Here's how the part is built. I have some questions about the finished solid (model axes, mm). Face numbers are marked on the shaded views. A direction names the side the tool comes from. Coordinates: 2 decimals unless noted, no trailing zeros. Write each loop counter-clockwise with the first axis right and the second up, starting at its lowest first coordinate (ties: lowest second). Pieces come first, ordered by that corner, then holes.
```python
from build123d import *

# Parameters (mm, degrees)
ESQUISSE1_R                        = 52
ESQUISSE1_R_2                      = 7
BOSS_EXTRU_1_DEPTH                 = 20
ESQUISSE2_W                        = 50
ESQUISSE2_H                        = 10
BOSS_EXTRU_2_DEPTH                 = 60
CONG_1_R                           = 25
ESQUISSE3_R                        = 6
ENL_V_MAT_EXTRU_1_DEPTH            = 40
R_P_TITION_CIRCULAIRE1_COUNT       = 2
CONG_1_OF_R_P_TITION_CIRCULAIRE1_R = 25
ESQUISSE5_R                        = 1.6
ENL_V_MAT_EXTRU_2_DEPTH            = 20
R_P_TITION_CIRCULAIRE2_COUNT       = 6
ESQUISSE6_R                        = 3
ENL_V_MAT_EXTRU_3_DEPTH            = 9
ENL_V_START                        = -10
ESQUISSE7_W                        = 80.1
ESQUISSE7_H                        = 5
ENL_V_MAT_EXTRU_4_DEPTH            = 45


with BuildPart() as part:
    # Esquisse1 → Boss.-Extru.1 (new body)
    with BuildSketch(Plane(origin=(0, 0, 0), x_dir=(1, 0, 0), z_dir=(0, 1, 0))):
        with Locations(Location((0, 0, 0), (0, 0, 270))):
            Circle(ESQUISSE1_R)
        with Locations(Location((0, 0, 0), (0, 0, 270))):
            Circle(ESQUISSE1_R_2, mode=Mode.SUBTRACT)
    extrude(amount=BOSS_EXTRU_1_DEPTH)

    # Esquisse2 → Boss.-Extru.2 (add)
    with BuildSketch(Plane(origin=(0, 20, 0), x_dir=(1, 0, 0), z_dir=(0, 1, 0))):
        with Locations((0, 25)):
            Rectangle(ESQUISSE2_W, ESQUISSE2_H)
    boss_extru_2 = extrude(amount=BOSS_EXTRU_2_DEPTH)

    # Congé1
    cong_1_edges = [part.edges().sort_by_distance(p)[0] for p in [
        (25, 80, -25),
        (-25, 80, -25),
    ]]
    fillet(cong_1_edges, radius=CONG_1_R - 0.0001)  # a hair under: the kernel refuses the full size

    # Esquisse3 → Enlèv. mat.-Extru.1 (cut)
    with BuildSketch(Plane(origin=(0, 0, -30), x_dir=(-1, 0, 0), z_dir=(0, 0, -1))):
        with Locations((0, 64)):
            Circle(ESQUISSE3_R)
    enl_v_mat_extru_1 = extrude(amount=-ENL_V_MAT_EXTRU_1_DEPTH, mode=Mode.SUBTRACT)

    # Répétition circulaire1: Boss.-Extru.2, Enlèv. mat.-Extru.1 ×2 about axis
    r_p_tition_circulaire1_axis = Axis((0, 0, 0), (0, 1, 0))
    add([boss_extru_2.rotate(r_p_tition_circulaire1_axis, i * 360 / R_P_TITION_CIRCULAIRE1_COUNT) for i in range(1, R_P_TITION_CIRCULAIRE1_COUNT)])
    add([enl_v_mat_extru_1.rotate(r_p_tition_circulaire1_axis, i * 360 / R_P_TITION_CIRCULAIRE1_COUNT) for i in range(1, R_P_TITION_CIRCULAIRE1_COUNT)], mode=Mode.SUBTRACT)

    # Congé1 of Répétition circulaire1
    cong_1_of_r_p_tition_circulaire1_edges = [part.edges().sort_by_distance(p)[0] for p in [
        (-25, 80, 25),
        (25, 80, 25),
    ]]
    fillet(cong_1_of_r_p_tition_circulaire1_edges, radius=CONG_1_OF_R_P_TITION_CIRCULAIRE1_R - 0.0001)  # a hair under: the kernel refuses the full size

    # Esquisse5 → Enlèv. mat.-Extru.2 (cut)
    with BuildSketch(Plane.XZ):
        with Locations(Location((0, 35, 0), (0, 0, 270))):
            Circle(ESQUISSE5_R)
    enl_v_mat_extru_2 = extrude(amount=-ENL_V_MAT_EXTRU_2_DEPTH, mode=Mode.SUBTRACT)

    # Répétition circulaire2: Enlèv. mat.-Extru.2 ×6 about axis
    r_p_tition_circulaire2_axis = Axis((0, 0, 0), (0, 1, 0))
    for i in range(1, R_P_TITION_CIRCULAIRE2_COUNT):
        add(enl_v_mat_extru_2.rotate(r_p_tition_circulaire2_axis, i * 360 / R_P_TITION_CIRCULAIRE2_COUNT), mode=Mode.SUBTRACT)

    # Esquisse6 → Enlèv. mat.-Extru.3 (cut)
    with BuildSketch(Plane(origin=(0, 20, 0), x_dir=(1, 0, 0), z_dir=(0, 1, 0))):
        with Locations(Location((30.310889132, 17.5, 0), (0, 0, 270))):
            Circle(ESQUISSE6_R)
        with Locations(Location((30.310889132, -17.5, 0), (0, 0, 270))):
            Circle(ESQUISSE6_R)
        with Locations(Location((0, -35, 0), (0, 0, 270))):
            Circle(ESQUISSE6_R)
        with Locations(Location((-30.310889132, -17.5, 0), (0, 0, 270))):
            Circle(ESQUISSE6_R)
        with Locations(Location((-30.310889132, 17.5, 0), (0, 0, 270))):
            Circle(ESQUISSE6_R)
        with Locations(Location((0, 35, 0), (0, 0, 270))):
            Circle(ESQUISSE6_R)
    extrude(amount=-ENL_V_MAT_EXTRU_3_DEPTH, mode=Mode.SUBTRACT)

    # Esquisse7 → Enlèv. mat.-Extru.4 (cut)
    with BuildSketch(Plane.XY.offset(ENL_V_START)):
        with Locations((0, 12.5)):
            Rectangle(ESQUISSE7_W, ESQUISSE7_H)
    extrude(amount=-ENL_V_MAT_EXTRU_4_DEPTH, mode=Mode.SUBTRACT)


solid = part.part
```
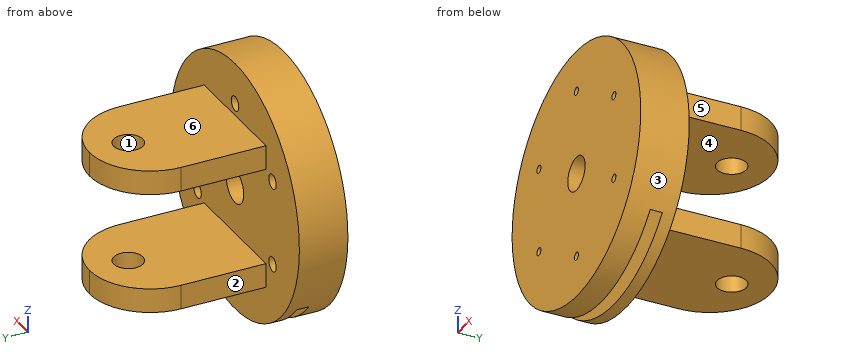
1) On a 3-axis mill with a long thin cutter (end or side, diameter ignored), from which of +Z, -Z, +X, -X, +Y, -Y can I reach the whole of each face in a straight line? I mean the marked faces 4, 5 and 6. Say none if no direction works.
Values follow:
face 4: +X, -X, +Y
face 5: +Z, -Z, +X, +Y
face 6: +Z, +X, -X, +Y
2) We'd pull the mould along X, two halves only. Please class the marked faces 1, 2 and 3: pulls with the +X half, pulls with the -X half, needs draft (parallel to the pull), parting line crosses it, or undercut.
Values follow:
face 1: undercut
face 2: pulls with the -X half
face 3: parting line crosses it
3) Imagine slicing it at D-D on z = 10.5. Please give me the cut outline in (x, y), then the cut area to 3 significant figures.
Values follow:
outline: (-50.93, 0) - (50.93, 0) - (50.93, 20) - (-50.93, 20) - close
area: 2,040 mm2
4) I need wall thicknesses on probe 1 along Z at (x, y) = (-16, 25.5); probe 2 along Y at (x, z) = (9, -38); probe 3 along X at (y, z) = (7, 17.5). Which ranges of each line are inside material? Lowest first, please.
Values follow:
probe 1: z = -30 to -20, 20 to 30
probe 2: y = 0 to 10, 15 to 20
probe 3: x = -48.97 to -31.91, -28.71 to 28.71, 31.91 to 48.97
5) Imagine slicing it at B-B on z = 0. Please give me the cut outline in (x, y).
Values follow:
outline: (-52, 0) - (-7, 0) - (-7, 20) - (-52, 20) - close; (7, 0) - (52, 0) - (52, 20) - (7, 20) - close
6) Imagine slicing it at C-C on z = -35. Please give me the cut outline in (x, y), then the cut area to 3 significant figures.
Values follow:
outline: (-38.46, 0) - (-1.6, 0) - (-1.6, 10) - (-38.46, 10) - close; (-38.46, 15) - (-3, 15) - (-3, 20) - (-38.46, 20) - close; (1.6, 0) - (38.46, 0) - (38.46, 10) - (1.6, 10) - close; (3, 15) - (38.46, 15) - (38.46, 20) - (3, 20) - close
area: 1,090 mm2
7) Will these pins go through, and if not, where does the flat tip stop? pin 1 (8 mm diameter, centred on x = -21.5, z = -28.5, fed in from -Y); pin 2 (3 mm diameter, centred on x = 20, y = 47, fed in from +Z); pin 3 (3.5 mm diameter, centred on x = -30.31, z = 17.5, fed in from +Y); pin 4 (8 mm diameter, centred on y = 44.5, z = -27, fed in from +X).
Values follow:
pin 1: stops at y = 0
pin 2: stops at z = 30
pin 3: stops at y = 11
pin 4: stops at x = 25
8) Imagine slicing it at A-A on y = 36. Please give me the cut outline in (x, z).
Values follow:
outline: (-25, -30) - (25, -30) - (25, -20) - (-25, -20) - close; (-25, 20) - (25, 20) - (25, 30) - (-25, 30) - close
